Design review of the part built by this model. Coordinates are the model's own, in mm. Face numbers are marked on the shaded views. Coordinates: 2 decimals unless noted, no trailing zeros. Write each loop counter-clockwise with the first axis right and the second up, starting at its lowest first coordinate (ties: lowest second). Pieces come first, ordered by that corner, then holes.
Q1. Add section A-A, the plane y = 26. Give the boundary of the cut face in (x, z), plus the area to 3 significant figures.
Q2. The part is to be moulded in two halves that separate along Y. For the marked faces 1, 2, 3 and 4, say which applies: +Y half, -Y half, draft (parallel to the pull), parting line (faces both ways), or undercut.
Q3. Add section B-B, the plane y = 15.5. Give the boundary of the cut face in (x, z), plus the area to 3 significant figures.
Q4. To check wall thickness, follow probe 1 along Z at (x, y) = (3, 26); probe 2 along X at (y, z) = (6, 10); probe 3 along Z at (x, y) = (-22, 3.9). State the ranges of each line that lie inside material, in increasing order.
Q5. Add section D-D, the plane z = -2.5. Give the boundary of the cut face in (x, y), plus the area to 3 significant figures.
Q6. Clearance check with flat-ended pins moving along their axes: pin 1 Ø5 at (x, z) = (-15, 13) entering from +Y; pin 2 Ø1.5 at (x, y) = (-8.5, 15) entering from +Z; pin 3 Ø2.5 at (x, z) = (-25.5, 11.5) entering from +Y. State where each tip first meets the part, or that it passes through.
Q7. Add section C-C, the plane x = -12. Give the boundary of the cut face in (y, z).
from build123d import *

# Parameters (mm, degrees)
CYLINDER005_R     = 6.5
CYLINDER005_DEPTH = 10
CYLINDER004_R     = 8.2
CYLINDER004_DEPTH = 5
BOX_W             = 10
BOX_H             = 26.4
BOX_DEPTH         = 26.4
FILLET_R          = 10
CYLINDER002_R     = 2.2
CYLINDER002_DEPTH = 20
ARRAY001_X_COUNT  = 2
ARRAY001_X_PITCH  = 44
PAD_DEPTH         = 20
PAD001_DEPTH      = 5


with BuildPart() as bring_holder_hole:
    # Cylinder005 → Cylinder005 (new body)
    with BuildSketch(Plane(origin=(0, 0, 0), x_dir=(0, 0, -1), z_dir=(1, 0, 0))):
        Circle(CYLINDER005_R)
    extrude(amount=CYLINDER005_DEPTH)


with BuildPart() as bring_holder_extract:
    # Cylinder004 → Cylinder004 (new body)
    with BuildSketch(Plane(origin=(0, 0, 0), x_dir=(0, 0, -1), z_dir=(1, 0, 0))):
        Circle(CYLINDER004_R)
    extrude(amount=CYLINDER004_DEPTH)

    # Fusion001: union bring holder hole
    add(bring_holder_hole.part)


with BuildPart() as bring_holder_cut:
    # Box → Box (new body)
    with BuildSketch(Plane(origin=(0, -13.2, -13.2), x_dir=(1, 0, 0), z_dir=(0, 0, 1))):
        with Locations((5, 13.2)):
            Rectangle(BOX_W, BOX_H)
    extrude(amount=BOX_DEPTH)

    # Fillet
    fillet_edges = [bring_holder_cut.edges().sort_by_distance(p)[0] for p in [
        (5, -13.2, -13.2),
        (5, 13.2, -13.2),
        (5, 13.2, 13.2),
    ]]
    fillet(fillet_edges, radius=FILLET_R)

    # Cut023015003: cut bring holder extract
    add(bring_holder_extract.part, mode=Mode.SUBTRACT)


with BuildPart() as bring_holder_cut_1:
    # Cut023015003 placement: moved
    add(bring_holder_cut.part.moved(Location((-5, 26, 7))))


with BuildPart() as bolt_hole_array001:
    # Cylinder002 → Cylinder002 (new body)
    with BuildSketch(Plane.XZ):
        Circle(CYLINDER002_R)
    extrude(amount=CYLINDER002_DEPTH)

    # Array001 X: bolt hole array001 ×2


with BuildPart() as bolt_hole_array001_1:
    add(bolt_hole_array001.part)
    with Locations(*[(i * ARRAY001_X_PITCH, 0, 0) for i in range(1, ARRAY001_X_COUNT)]):
        add(bolt_hole_array001.part)


with BuildPart() as bolt_hole_array001_2:
    # Array001 placement: moved
    add(bolt_hole_array001_1.part.moved(Location((-22, 20, 10))))


with BuildPart() as f_25_mm_16mm_bring_attachment_fusion:
    # Sketch → Pad (new body)
    with BuildSketch(Plane.XY):
        with BuildLine():
            ThreePointArc((12.611106, 1.5), (0, 12.7), (-12.611106, 1.5))
            Line((-22.7, 1.5), (-12.611106, 1.5))
            Line((-22.7, 1.5), (-22.7, 6.5))
            Line((-22.7, 6.5), (-21.463293, 6.5))
            Line((-21.463293, 6.5), (-13.988671, 10.84468))
            ThreePointArc((13.988671, 10.84468), (0, 17.7), (-13.988671, 10.84468))
            Line((13.988671, 10.84468), (21.463293, 6.5))
            Line((21.463293, 6.5), (22.7, 6.5))
            Line((22.7, 6.5), (22.7, 1.5))
            Line((12.611106, 1.5), (22.7, 1.5))
        make_face()
    extrude(amount=PAD_DEPTH)

    # Sketch001 → Pad001 (join)
    with BuildSketch(Plane.XZ.offset(-1.5)):
        with BuildLine():
            Line((-12.611106, 20), (-22.7, 20))
            ThreePointArc((-22.7, 20), (-27.649747, 17.949747), (-29.7, 13))
            Line((-29.7, 13), (-29.7, 7))
            ThreePointArc((-29.7, 7), (-27.649747, 2.050253), (-22.7, 0))
            Line((-12.611106, 0), (-22.7, 0))
            Line((-12.611106, 20), (-12.611106, 0))
        make_face()
        with BuildLine():
            Line((12.611106, 20), (22.7, 20))
            ThreePointArc((29.7, 13), (27.649747, 17.949747), (22.7, 20))
            Line((29.7, 13), (29.7, 7))
            ThreePointArc((22.7, 0), (27.649747, 2.050253), (29.7, 7))
            Line((22.7, 0), (12.611106, 0))
            Line((12.611106, 20), (12.611106, 0))
        make_face()
    extrude(amount=-PAD001_DEPTH)

    # Cut023015002: cut bolt hole array001
    add(bolt_hole_array001_2.part, mode=Mode.SUBTRACT)

    # Fusion002: union bring holder cut
    add(bring_holder_cut_1.part)


solid = f_25_mm_16mm_bring_attachment_fusion.part
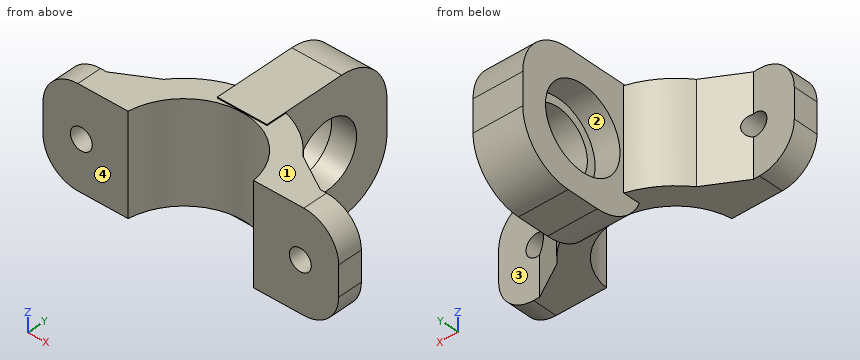
Here are the results:
1. outline: (-5, -6.2) - (5, -6.2) - (5, 0.5) - (0, 0.5) - (0, -1.2) - (-5, -1.2) - close; (-5, 15.2) - (0, 15.2) - (0, 13.5) - (5, 13.5) - (5, 20.2) - (-5, 20.2) - close
1. area: 117 mm2
2. face 1: draft
2. face 2: undercut
2. face 3: +Y half
2. face 4: -Y half
3. outline: (-8.55, 0) - (-5, 0) - (-5, -3.03) - (5, -3.03) - (5, 0) - (8.55, 0) - (8.55, 20) - (5, 20) - (5, 20.2) - (-5, 20.2) - (-5, 20) - (-8.55, 20) - close
3. area: 374 mm2
4. probe 1: z = -6.2 to 0.5, 13.5 to 20.2
4. probe 2: x = -29.7 to -24.2, -19.8 to -11.19, 11.19 to 19.8, 24.2 to 29.7
4. probe 3: z = 0 to 7.8, 12.2 to 20
5. outline: (-5, 15.03) - (5, 15.03) - (5, 36.97) - (-5, 36.97) - close
5. area: 219 mm2
6. pin 1: stops at y = 12.53
6. pin 2: stops at z = 20
6. pin 3: stops at y = 6.5
7. outline: (4.16, 0) - (13.01, 0) - (13.01, 20) - (4.16, 20) - close
